Can you work these out from the model? Positions are in its coordinate system, mm. A direction names the side the tool comes from. Give positions to 0.01 mm unless a question says otherwise; leave off trailing zeros. Loops run counter-clockwise (first coordinate to the right, second up) from the corner with the lowest first, then second, coordinate; pieces in that order, holes last.
from build123d import *

# Parameters (mm, degrees)
BOSS_EXTRUDE1_DEPTH = 3


with BuildPart() as part:
    # Sketch4 → Boss-Extrude1 (new body, symmetric)
    with BuildSketch(Plane.XY):
        with BuildLine():
            Line((-49.569635322, 11.648391942), (-5.913243351, 22.914313825))
            ThreePointArc((-5.913243351, 22.914313825), (23.665, 0), (-5.913243351, -22.914313825))
            Line((-5.913243351, -22.914313825), (-49.569635322, -11.648391942))
            ThreePointArc((-49.569635322, -11.648391942), (-58.593663739, 0), (-49.569635322, 11.648391942))
        make_face()
        with BuildLine():
            Line((-49.409716634, 11.028693618), (-5.753324663, 22.294615501))
            ThreePointArc((-5.753324663, 22.294615501), (23.025, 0), (-5.753324663, -22.294615501))
            Line((-5.753324663, -22.294615501), (-49.409716634, -11.028693618))
            ThreePointArc((-49.409716634, -11.028693618), (-57.953663739, 0), (-49.409716634, 11.028693618))
        make_face(mode=Mode.SUBTRACT)
    extrude(amount=BOSS_EXTRUDE1_DEPTH, both=True)


solid = part.part
(1) Please list where these lines run through material, in increasing order: probe 1 along Y at (x, z) = (0, 1.5) (3 decimals); probe 2 along X at (y, z) = (6.5, -0.8); probe 3 along Y at (x, z) = (-8.5, -0.05).
Returned:
probe 1: y = -23.665 to -23.025, 23.025 to 23.665
probe 2: x = -56.69 to -55.92, 22.09 to 22.75
probe 3: y = -22.25 to -21.59, 21.59 to 22.25
(2) Suppose I cut it at A-A on y = 0. List the corners of the cut face in (x, z) for me (3 decimals).
Returned:
outline: (-58.594, -3) - (-57.954, -3) - (-57.954, 3) - (-58.594, 3) - close; (23.025, -3) - (23.665, -3) - (23.665, 3) - (23.025, 3) - close
(3) Suppose I cut it at B-B on z = -0.4. List the corners of the cut face in (x, y) for me (3 decimals).
Returned:
outline: (-49.57, -11.648) - (-5.913, -22.914) arc R23.665 ccw (long way) to (-5.913, 22.914) - (-49.57, 11.648) arc R12.03 ccw to start; hole (-49.41, -11.029) - (-5.753, -22.295) arc R23.025 ccw (long way) to (-5.753, 22.295) - (-49.41, 11.029) arc R11.39 ccw to start
(4) Thinking about a two-plate mould opening in Y: for faces 3 (the flat face through (-28.05, 17.2, 0.04)), 4 (the cylindrical face through (-57.95, -0.21, 0.04)), 5 (the flat face through (-27.44, -17.36, 0.04)), which applies, pulls with the +Y half, pulls with the -Y half, needs draft (parallel to the pull), parting line crosses it, or undercut?
Returned:
face 3: pulls with the +Y half
face 4: undercut
face 5: pulls with the -Y half
(5) Will this pin go through, and if not, where does the flat tip stop? P1, Ø3, axis at x = -47, z = 2, coming from the -Y side.
Returned:
P1: stops at y = -12.7
(6) Suppose I cut it at C-C on x = 0. List the corners of the cut face in (y, z) for me (3 decimals).
Returned:
outline: (-23.665, -3) - (-23.025, -3) - (-23.025, 3) - (-23.665, 3) - close; (23.025, -3) - (23.665, -3) - (23.665, 3) - (23.025, 3) - close
(7) Which directions (+Z, -Z, +X, -X, +Y, -Y) give clear straight access to the entire face, cutting with the end or side of a thin tool? Please do faces 1 (the cylindrical face through (-58.59, -0.22, 0.04)), 2 (the flat face through (-27.28, -16.74, 0.04)).
Returned:
face 1: +Z, -Z, -X
face 2: +Z, -Z
